from build123d import *

# Parameters (mm, degrees)
CYLINDER1890_R               = 1.5
CYLINDER1890_DEPTH           = 20
CYLINDER1890_PLACEMENT_ANGLE = -112.5
CYLINDER1891_R               = 1.5
CYLINDER1891_DEPTH           = 20
CYLINDER1891_PLACEMENT_ANGLE = 112.5
CYLINDER1892_R               = 1.5
CYLINDER1892_DEPTH           = 20
CYLINDER1892_PLACEMENT_ANGLE = 112.5
CYLINDER1893_R               = 1.5
CYLINDER1893_DEPTH           = 20
CYLINDER1893_PLACEMENT_ANGLE = -112.5
CYLINDER1885_R               = 3
CYLINDER1885_DEPTH           = 3
CYLINDER1885_PLACEMENT_ANGLE = -112.5
CYLINDER1894_R               = 3
CYLINDER1894_DEPTH           = 3
CYLINDER1894_PLACEMENT_ANGLE = 112.5
CYLINDER1895_R               = 3
CYLINDER1895_DEPTH           = 3
CYLINDER1895_PLACEMENT_ANGLE = 112.5
CYLINDER1884_R               = 3
CYLINDER1884_DEPTH           = 3
CYLINDER1884_PLACEMENT_ANGLE = -112.5
BOX748_W                     = 26
BOX748_H                     = 44
BOX748_DEPTH                 = 2


with BuildPart() as obj1:
    # Cylinder1890 → Cylinder1890 (new body)
    with BuildSketch(Plane.XY):
        Circle(CYLINDER1890_R)
    extrude(amount=CYLINDER1890_DEPTH)


with BuildPart() as obj1_1:
    # Cylinder1890 placement: moved
    add(obj1.part.moved(Location((-8, 34, 51))).rotate(Axis((-8, 34, 51), (0, 0, 1)), CYLINDER1890_PLACEMENT_ANGLE))


with BuildPart() as obj2:
    # Cylinder1891 → Cylinder1891 (new body)
    with BuildSketch(Plane.XY):
        Circle(CYLINDER1891_R)
    extrude(amount=CYLINDER1891_DEPTH)


with BuildPart() as obj2_1:
    # Cylinder1891 placement: moved
    add(obj2.part.moved(Location((8, 62, 51))).rotate(Axis((8, 62, 51), (0, 0, -1)), CYLINDER1891_PLACEMENT_ANGLE))


with BuildPart() as obj3:
    # Cylinder1892 → Cylinder1892 (new body)
    with BuildSketch(Plane.XY):
        Circle(CYLINDER1892_R)
    extrude(amount=CYLINDER1892_DEPTH)


with BuildPart() as obj3_1:
    # Cylinder1892 placement: moved
    add(obj3.part.moved(Location((-8, 62, 51))).rotate(Axis((-8, 62, 51), (0, 0, -1)), CYLINDER1892_PLACEMENT_ANGLE))


with BuildPart() as compound848:
    # Cylinder1893 → Cylinder1893 (new body)
    with BuildSketch(Plane.XY):
        Circle(CYLINDER1893_R)
    extrude(amount=CYLINDER1893_DEPTH)


with BuildPart() as compound848_1:
    # Cylinder1893 placement: moved
    add(compound848.part.moved(Location((8, 34, 51))).rotate(Axis((8, 34, 51), (0, 0, 1)), CYLINDER1893_PLACEMENT_ANGLE))

    # Compound848: union obj1, obj2, obj3
    add(obj1_1.part)
    add(obj2_1.part)
    add(obj3_1.part)


with BuildPart() as compound848_2:
    # Compound848 placement: moved
    add(compound848_1.part.moved(Location((0, -94, -180))))


with BuildPart() as obj4:
    # Cylinder1885 → Cylinder1885 (new body)
    with BuildSketch(Plane.XY):
        Circle(CYLINDER1885_R)
    extrude(amount=CYLINDER1885_DEPTH)


with BuildPart() as obj4_1:
    # Cylinder1885 placement: moved
    add(obj4.part.moved(Location((-8, 34, 51))).rotate(Axis((-8, 34, 51), (0, 0, 1)), CYLINDER1885_PLACEMENT_ANGLE))


with BuildPart() as obj5:
    # Cylinder1894 → Cylinder1894 (new body)
    with BuildSketch(Plane.XY):
        Circle(CYLINDER1894_R)
    extrude(amount=CYLINDER1894_DEPTH)


with BuildPart() as obj5_1:
    # Cylinder1894 placement: moved
    add(obj5.part.moved(Location((8, 62, 51))).rotate(Axis((8, 62, 51), (0, 0, -1)), CYLINDER1894_PLACEMENT_ANGLE))


with BuildPart() as obj6:
    # Cylinder1895 → Cylinder1895 (new body)
    with BuildSketch(Plane.XY):
        Circle(CYLINDER1895_R)
    extrude(amount=CYLINDER1895_DEPTH)


with BuildPart() as obj6_1:
    # Cylinder1895 placement: moved
    add(obj6.part.moved(Location((-8, 62, 51))).rotate(Axis((-8, 62, 51), (0, 0, -1)), CYLINDER1895_PLACEMENT_ANGLE))


with BuildPart() as compound847:
    # Cylinder1884 → Cylinder1884 (new body)
    with BuildSketch(Plane.XY):
        Circle(CYLINDER1884_R)
    extrude(amount=CYLINDER1884_DEPTH)


with BuildPart() as compound847_1:
    # Cylinder1884 placement: moved
    add(compound847.part.moved(Location((8, 34, 51))).rotate(Axis((8, 34, 51), (0, 0, 1)), CYLINDER1884_PLACEMENT_ANGLE))

    # Compound847: union obj4, obj5, obj6
    add(obj4_1.part)
    add(obj5_1.part)
    add(obj6_1.part)


with BuildPart() as compound847_2:
    # Compound847 placement: moved
    add(compound847_1.part.moved(Location((0, -94, -183))))


with BuildPart() as cut687:
    # Box748 → Box748 (new body)
    with BuildSketch(Plane(origin=(-13, -66, -130), x_dir=(1, 0, 0), z_dir=(0, 0, 1))):
        with Locations((13, 22)):
            Rectangle(BOX748_W, BOX748_H)
    extrude(amount=BOX748_DEPTH)

    # Cut686: cut Compound847
    add(compound847_2.part, mode=Mode.SUBTRACT)

    # Cut687: cut Compound848
    add(compound848_2.part, mode=Mode.SUBTRACT)


with BuildPart() as cut687_1:
    # Cut687 placement: moved
    add(cut687.part.moved(Location((0, 0, 1))))


solid = cut687_1.part
For this review, take the finished solid that the model builds, in its own axes (mm). A direction names the side the tool comes from. Give positions to 0.01 mm unless a question says otherwise; leave off trailing zeros. Order: outer loops, then holes, each group sorted by start corner. A loop starts at its lowest first (then second) coordinate and runs counter-clockwise, first axis right, second up. Notation, with made-up numbers: (-39.5, -9) - (-10.5, -9) arc R24 cw to (-10.5, 19) - close; hole circle Ø3 at (82.25, 75). An arc over 180 degrees is marked (long way). Answer as a JSON object with one key per item and string values. Group by question number.
Item 1: Take a section at C-C on z = -127.55. Give the boundary of the cut face in (x, y).
Item 2: Take a section at B-B on y = -60. Give the boundary of the cut face in (x, z).
Item 3: Draft analysis for pull direction Z (two halves, no side actions). For faces 1 (the flat face through (0, -44, -127)), 2 (the flat face through (-8, -58, -128)), 3 (the flat face through (0, -66, -128)), state which applies: pulls with the +Z half, pulls with the -Z half, needs draft (parallel to the pull), parting line crosses it, or undercut.
Item 4: Clearance check with flat-ended pins moving along their axes: pin 1 Ø2.5 at (x, y) = (8, -60) entering from +Z; pin 2 Ø3.5 at (x, y) = (-8, -32) entering from -Z. State where each tip first meets the part, or that it passes through.
Item 5: Take a section at A-A on x = 8. Give the boundary of the cut face in (y, z).
Item 6: Machinability: for faces 4 (the flat face through (0, -44, -129)), 5 (the flat face through (8, -58, -128)), which of the approach directions +Z, -Z, +X, -X, +Y, -Y give a long, thin tool a straight path to every point of the face, cutting with its end or side? Answer none if there is none.
Item 7: Wall thickness on line 1 along Y through (x, z) = (-8, -128.65); line 2 along Y through (x, z) = (-8, -127.35); line 3 along X through (y, z) = (-60, -127.45): over which ranges is each line inside the solid? List them lowest first.
Reported:
{
 "1": {"outline": "(-13, -66) - (13, -66) - (13, -22) - (-13, -22) - close; hole circle Ø3 at (-8, -60); hole circle Ø3 at (-8, -32); hole circle Ø3 at (8, -60); hole circle Ø3 at (8, -32)"},
 "2": {"outline": "(-13, -129) - (-11, -129) - (-11, -128) - (-9.5, -128) - (-9.5, -127) - (-13, -127) - close; (-6.5, -128) - (-5, -128) - (-5, -129) - (5, -129) - (5, -128) - (6.5, -128) - (6.5, -127) - (-6.5, -127) - close; (9.5, -128) - (11, -128) - (11, -129) - (13, -129) - (13, -127) - (9.5, -127) - close"},
 "3": {"face 1": "pulls with the +Z half", "face 2": "pulls with the -Z half", "face 3": "needs draft"},
 "4": {"pin 1": "through", "pin 2": "z = -128"},
 "5": {"outline": "(-66, -129) - (-63, -129) - (-63, -128) - (-61.5, -128) - (-61.5, -127) - (-66, -127) - close; (-58.5, -128) - (-57, -128) - (-57, -129) - (-35, -129) - (-35, -128) - (-33.5, -128) - (-33.5, -127) - (-58.5, -127) - close; (-30.5, -128) - (-29, -128) - (-29, -129) - (-22, -129) - (-22, -127) - (-30.5, -127) - close"},
 "6": {"face 4": "-Z, +X, -X, +Y, -Y", "face 5": "-Z"},
 "7": {"line 1": "-66 to -63, -57 to -35, -29 to -22", "line 2": "-66 to -61.5, -58.5 to -33.5, -30.5 to -22", "line 3": "-13 to -9.5, -6.5 to 6.5, 9.5 to 13"}
}
